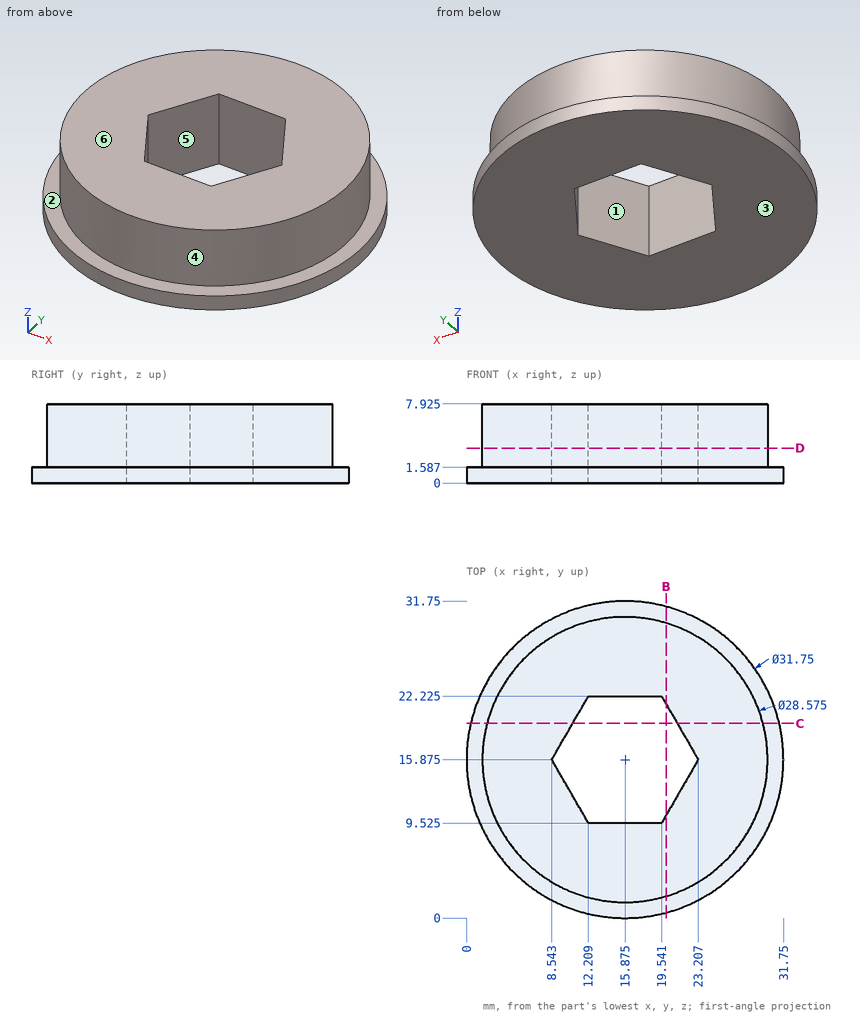
Print and shaded views of the part. All mm, measured from the part's lowest x, y and z. A direction names the side the tool comes from. Coordinates: 2 decimals unless noted, no trailing zeros. Loops run counter-clockwise (first coordinate to the right, second up) from the corner with the lowest first, then second, coordinate; pieces in that order, holes last. Notation, with made-up numbers: (38.5, -27) -> (57.5, -27) arc R10 cw to (57.5, -16) -> close; hole circle Ø5 at (55, 53). An arc over 180 degrees is marked (long way). Use one line per item in the form item = value. Start each with the question number.
(1) Cut at B-B on x = 20. Give the cut face in (y, z) (1 decimal).
(2) Tool access for the marked faces 1, 2 and 3: list every direction of +Z, -Z, +X, -X, +Y, -Y with a clear straight run to the whole face (end or side of a thin tool).
(3) Cut at D-D on z = 3.5. Give the cut face in (x, y) (1 decimal).
(4) Flat gauge pins, fed straight in: pin 1 (3 mm diameter, centred on y = 19.5, z = 4.5, fed in from -X); pin 2 (3 mm diameter, centred on x = 11.5, z = 3, fed in from +Y). Where does each tip first touch, or does it go through?
(5) Pull direction Y, two halves, no side cores. Call the marked faces 4, 5 and 6: pulls with the +Y half, pulls with the -Y half, needs draft (parallel to the pull), parting line crosses it, or undercut.
(6) Cut at C-C on y = 19.5. Give the cut face in (x, z) (1 decimal).
(7) Probe probe 1 along Y at (x, z) = (15.5, 4.75) (1 decimal); probe 2 along Y at (x, z) = (22, 5.5) (1 decimal); probe 3 along X at (y, z) = (17.5, 2). List the from-to ranges inside material, lowest first. Write a range as from..to.
Values:
q1.outline = (0.5, 0) -> (10.3, 0) -> (10.3, 7.9) -> (2.2, 7.9) -> (2.2, 1.6) -> (0.5, 1.6) -> close; (21.4, 0) -> (31.2, 0) -> (31.2, 1.6) -> (29.6, 1.6) -> (29.6, 7.9) -> (21.4, 7.9) -> close
q2.face_1 = +Z, -Z
q2.face_2 = +Z
q2.face_3 = -Z, +X, -X, +Y, -Y
q3.outline = circle Ø28.6 at (15.9, 15.9); hole (8.5, 15.9) -> (12.2, 9.5) -> (19.5, 9.5) -> (23.2, 15.9) -> (19.5, 22.2) -> (12.2, 22.2) -> close
q4.pin_1 = 1.75
q4.pin_2 = 31.27
q5.face_4 = parting line crosses it
q5.face_5 = undercut
q5.face_6 = needs draft
q6.outline = (0.4, 0) -> (10.6, 0) -> (10.6, 7.9) -> (2.1, 7.9) -> (2.1, 1.6) -> (0.4, 1.6) -> close; (21.1, 0) -> (31.3, 0) -> (31.3, 1.6) -> (29.7, 1.6) -> (29.7, 7.9) -> (21.1, 7.9) -> close
q7.probe_1 = 1.6..9.5, 22.2..30.2
q7.probe_2 = 3..13.8, 18..28.8
q7.probe_3 = 1.68..9.48, 22.27..30.07
